Autodesk Inventor part; units mm, degrees
ref_plane "body_to_teeth_XY" through (0, 0, 0) normal (1, 0, 0) x (0, 0, -1)
ref_plane "body_to_teeth_YZ" through (0, 0, 0) normal (0, 0, -1) x (0, 1, 0)
ref_plane "body_to_teeth_ZX" through (0, 0, 0) normal (0, 1, 0) x (1, 0, 0)
sketch "Sketch_11" plane through (0, 0, 0) normal (0, 0, 1) x (1, 0, 0)
  line L0 (20, 0) -> (0, 0)
  line L1 (0, 0) -> (0, 34)
  line L2 (0, 34) -> (0.5359, 36)
  line L3 (0.5359, 36) -> (9.4641, 36)
  line L4 (9.4641, 36) -> (10, 34)
  line L5 (10, 34) -> (10, 20)
  line L6 (10, 20) -> (19.7, 20)
  line L7 (19.7, 20) -> (20, 19.7)
  line L8 (20, 19.7) -> (20, 0)
  line L9 (20, 0) -> (0, 0)
revolve "Revolution1" add sketch "Sketch_11" angle 360 about axis through (20, 0, 0) along (1, 0, 0)
sketch "Sketch_2" plane through (0, 0, 0) normal (1, 0, 0) x (0, 1, 0)
  circle A0 centre (0, 0) radius 41
  circle A1 centre (0, 0) radius 22.5
extrude "Extrusion1" cut sketch "Sketch_2" along normal blind 10
sketch "_____1" plane through (0, 0, 0) normal (0, 0, 1) x (1, 0, 0)
  line L0 (40, 0) -> (-40, 0)
  line L1 (0, 0) -> (0, 5.3)
  line L2 (0, 5.3) -> (0.3, 5)
  line L3 (0.3, 5) -> (19.7, 5)
  line L4 (19.7, 5) -> (20, 5.3)
  line L5 (20, 5.3) -> (20, 0)
  line L6 (20, 0) -> (0, 0)
revolve "Revolution2" cut sketch "_____1" angle 360 about axis through (40, 0, 0) along (1, 0, 0)
sketch "Sketch_3" plane through (0, 0, 0) normal (0, 0, 1) x (1, 0, 0)
  line L0 (15, 0) -> (15, 21)
  line L1 (15, 21) -> (17, 21)
  line L2 (17, 21) -> (17, 20)
  line L3 (17, 20) -> (16.621, 19.621)
  line L4 (16.621, 19.621) -> (16.621, 0)
  line L5 (16.621, 0) -> (15, 0)
  line L6 (15, 0) -> (15, 21)
revolve "Revolution3" cut sketch "Sketch_3" angle 360 about axis through (15, 0, 0) along (0, -1, 0)
thread "Thread1"
sketch "Sketch_5" plane through (0, 0, 0) normal (1, 0, 0) x (0, 1, 0)
  line L0 (6.6, 2) -> (0, 2)
  line L1 (0, 2) -> (0, -2)
  line L2 (0, -2) -> (6.6, -2)
  arc A0 (6.6, -2) -> (6.8, -1.8) centre (6.6, -1.8) ccw
  line L3 (6.8, -1.8) -> (6.8, 1.8)
  arc A1 (6.8, 1.8) -> (6.6, 2) centre (6.6, 1.8) ccw
extrude "Extrusion2" cut sketch "Sketch_5" along normal blind 20
ref_plane "body_to_teeth_XY" through (0, 0, 0) normal (1, 0, 0) x (0, 0, -1)
ref_plane "body_to_teeth_YZ" through (0, 0, 0) normal (0, 0, -1) x (0, 1, 0)
ref_plane "body_to_teeth_ZX" through (0, 0, 0) normal (0, 1, 0) x (1, 0, 0)
ref_plane "screw1_XY" through (15, 20, 0) normal (0, -1, 0) x (1, 0, 0)
ref_plane "screw1_YZ" through (15, 20, 0) normal (1, 0, 0) x (0, 0, 1)
ref_plane "screw1_ZX" through (15, 20, 0) normal (0, 0, 1) x (0, -1, 0)
ref_plane "screw2_XY" through (15, 0, -20) normal (0, 0, -1) x (1, 0, 0)
ref_plane "screw2_YZ" through (15, 0, -20) normal (1, 0, 0) x (0, -1, 0)
ref_plane "screw2_ZX" through (15, 0, -20) normal (0, -1, 0) x (0, 0, -1)
ref_plane "screw3_XY" through (15, -10, -17.3205) normal (0, -0.5, -0.866) x (1, 0, 0)
ref_plane "screw3_YZ" through (15, -10, -17.3205) normal (1, 0, 0) x (0, -0.866, 0.5)
ref_plane "screw3_ZX" through (15, -10, -17.3205) normal (0, -0.866, 0.5) x (0, -0.5, -0.866)
properties part number "GEYK1.0-70-10-B-10K.0_b"
Input: part model. Units: mm. Frame: model coordinates. A direction names the side the tool comes from. Coordinates: 2 decimals unless noted, no trailing zeros. Loops run counter-clockwise (first coordinate to the right, second up) from the corner with the lowest first, then second, coordinate; pieces in that order, holes last. Notation, with made-up numbers: (35, 17.25) - (88, 17.25) arc R16 cw to (88, 40.25) - close; hole circle Ø10 at (29, 26). An arc over 180 degrees is marked (long way). Answer in a Markdown table with one row per item.
(1) Set-up query: faces 1 (the face through (10, 6, -2)), 2 (the face through (10, -20.1, -1.6)), 3 (the face through (16.546, 13.121, 0.487)). Return all of +Z, -Z, +X, -X, +Y, -Y with unobstructed straight access to the full face (end or side cutting, diameter ignored); none if empty.
Model answer:
| item | result |
|---|---|
| face 1 | +X, -X |
| face 2 | +X |
| face 3 | +Y |
(2) Mould query, pull axis Y, two halves, no side actions, for faces 4 (the face through (0.181, -5.115, -0.197)), 5 (the face through (0, 5, -5)), 6 (the face through (14.918, -4.336, -19.524)). Classes: pulls with the +Y half, pulls with the -Y half, needs draft (parallel to the pull), parting line crosses it, or undercut.
Model answer:
| item | result |
|---|---|
| face 4 | undercut |
| face 5 | needs draft |
| face 6 | parting line crosses it |
(3) Cut plane B-B on y = 0. Output: boundary loops of the cut face in (x, z).
Model answer:
| item | result |
|---|---|
| outline | (0, -22.5) - (10, -22.5) - (10, -20) - (19.7, -20) - (20, -19.7) - (20, -5.3) - (19.7, -5) - (0.3, -5) - (0, -5.3) - close; (0, 5.3) - (0.3, 5) - (19.7, 5) - (20, 5.3) - (20, 19.7) - (19.7, 20) - (10, 20) - (10, 22.5) - (0, 22.5) - close |
(4) Cut plane C-C on z = 0. Output: boundary loops of the cut face in (x, y).
Model answer:
| item | result |
|---|---|
| outline | (0, -22.5) - (10, -22.5) - (10, -20) - (19.7, -20) - (20, -19.7) - (20, -5.3) - (19.7, -5) - (0.3, -5) - (0, -5.3) - close; (0, 6.8) - (13.38, 6.8) - (13.38, 19.62) - (13, 20) - (10, 20) - (10, 22.5) - (0, 22.5) - close; (16.62, 6.8) - (20, 6.8) - (20, 19.7) - (19.7, 20) - (17, 20) - (16.62, 19.62) - close |
(5) Pin query (flat end, axial travel): P1, Ø5, axis at x = 11, z = -14, coming from the -Y side; P2, Ø2, axis at x = 13, y = 5.5, coming from the -Z side; P3, Ø3, axis at y = 16, z = -0.5, coming from the -X side; P4, Ø1, axis at x = 8.5, y = 5.5, coming from the +Z side. Return the tip coordinate at first contact, or that it passes through.
Model answer:
| item | result |
|---|---|
| P1 | stops at y = -19.21 |
| P2 | stops at z = -19.49 |
| P3 | stops at x = 0 |
| P4 | stops at z = 21.94 |
(6) Cut plane D-D on x = 15. Output: boundary loops of the cut face in (y, z), plus the area to 3 significant figures.
Model answer:
| item | result |
|---|---|
| outline | (4.58, -2) arc R5 cw (long way) to (4.58, 2) - (6.6, 2) arc R0.2 cw to (6.8, 1.8) - (6.8, 1.62) - (19.62, 1.62) - (19.91, 1.91) arc R20 ccw (long way) to (19.91, -1.91) - (19.62, -1.62) - (6.8, -1.62) - (6.8, -1.8) arc R0.2 cw to (6.6, -2) - close |
| area | 1,130 mm² |
(7) Material intervals for L1, parallel to Z at x = 8.5, y = 0; L2, parallel to Z at x = 10.75, y = 0; L3, parallel to X at y = 9.5, z = -18, sorted ascending. Write a range as from..to.
Model answer:
| item | result |
|---|---|
| L1 | z = -22.5..-5, 5..22.5 |
| L2 | z = -20..-5, 5..20 |
| L3 | x = 0..10 |
(8) Cut plane A-A on x = 18.5. Output: boundary loops of the cut face in (y, z), plus the area to 3 significant figures.
Model answer:
| item | result |
|---|---|
| outline | circle Ø40 at (0, 0); hole (4.58, -2) - (6.6, -2) arc R0.2 ccw to (6.8, -1.8) - (6.8, 1.8) arc R0.2 ccw to (6.6, 2) - (4.58, 2) arc R5 ccw (long way) to start |
| area | 1,170 mm² |
